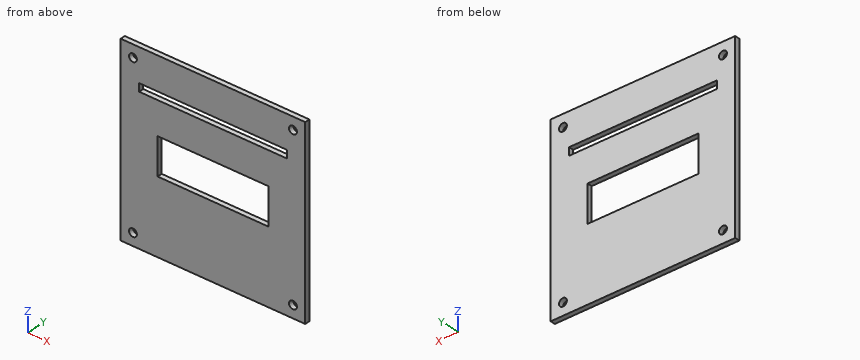
```python
from build123d import *

# Parameters (mm, degrees)
SKETCH1_W           = 75
SKETCH1_H           = 75
SKETCH1_R           = 1.6
BOSS_EXTRUDE1_DEPTH = 2
SKETCH2_W           = 45
SKETCH2_H           = 15
CUT_EXTRUDE1_DEPTH  = 10
SKETCH3_W           = 30
SKETCH3_H           = 3.2
CUT_EXTRUDE2_DEPTH  = 10


with BuildPart() as part:
    # Sketch1 → Boss-Extrude1 (new body)
    with BuildSketch(Plane(origin=(0, 0, 0), x_dir=(1, 0, 0), z_dir=(0, 1, 0))):
        Rectangle(SKETCH1_W, SKETCH1_H)
        with Locations(Location((-32.5, 32.5, 0), (0, 0, 270))):
            Circle(SKETCH1_R, mode=Mode.SUBTRACT)
        with Locations(Location((-32.5, -32.5, 0), (0, 0, 270))):
            Circle(SKETCH1_R, mode=Mode.SUBTRACT)
        with Locations(Location((32.5, 32.5, 0), (0, 0, 270))):
            Circle(SKETCH1_R, mode=Mode.SUBTRACT)
        with Locations(Location((32.5, -32.5, 0), (0, 0, 270))):
            Circle(SKETCH1_R, mode=Mode.SUBTRACT)
    extrude(amount=BOSS_EXTRUDE1_DEPTH)

    # Sketch2 → Cut-Extrude1 (cut)
    with BuildSketch(Plane.XZ):
        Rectangle(SKETCH2_W, SKETCH2_H)
    extrude(amount=-CUT_EXTRUDE1_DEPTH, mode=Mode.SUBTRACT)

    # Sketch3 → Cut-Extrude2 (cut)
    with BuildSketch(Plane.XZ):
        with Locations((-15, 22.5)):
            Rectangle(SKETCH3_W, SKETCH3_H)
        with Locations((15, 22.5)):
            Rectangle(SKETCH3_W, SKETCH3_H)
    extrude(amount=-CUT_EXTRUDE2_DEPTH, mode=Mode.SUBTRACT)


solid = part.part
```
Read the model definition and answer for the solid it produces. Units are mm, in the model's axes. Give positions to 0.01 mm unless a question says otherwise; leave off trailing zeros. Loops run counter-clockwise (first coordinate to the right, second up) from the corner with the lowest first, then second, coordinate; pieces in that order, holes last.
Item 1: Find the intervals of material crossed by line 1 along Z through (x, y) = (-22, 1.55); line 2 along X through (y, z) = (0.65, -32.5); line 3 along X through (y, z) = (1.5, 21), in increasing order.
Item 2: The part is cut by section D-D (x = 24). Write down the section's boundary in (y, z), and give its area (3 significant figures).
Item 3: The part is cut by section B-B (x = -14.5). Write down the section's boundary in (y, z), and give its area (3 significant figures).
Item 4: This flat-tipped pin is pushed along its axis until it touches: pin 1 Ø1.9 at (x, z) = (-32.5, 32.5) entering from -Y. Where does it stop, or does it pass through?
Item 5: The part is cut by section C-C (z = 32.5). Write down the section's boundary in (x, y), and give its area (3 significant figures).
Item 6: The part is cut by section A-A (z = 6). Write down the section's boundary in (x, y).
Taken from the geometry:
1. line 1: z = -37.5 to -7.5, 7.5 to 20.9, 24.1 to 37.5
1. line 2: x = -37.5 to -34.1, -30.9 to 30.9, 34.1 to 37.5
1. line 3: x = -37.5 to -30, 30 to 37.5
2. outline: (0, -37.5) - (2, -37.5) - (2, 20.9) - (0, 20.9) - close; (0, 24.1) - (2, 24.1) - (2, 37.5) - (0, 37.5) - close
2. area: 144 mm2
3. outline: (0, -37.5) - (2, -37.5) - (2, -7.5) - (0, -7.5) - close; (0, 7.5) - (2, 7.5) - (2, 20.9) - (0, 20.9) - close; (0, 24.1) - (2, 24.1) - (2, 37.5) - (0, 37.5) - close
3. area: 114 mm2
4. pin 1: passes through
5. outline: (-37.5, 0) - (-34.1, 0) - (-34.1, 2) - (-37.5, 2) - close; (-30.9, 0) - (30.9, 0) - (30.9, 2) - (-30.9, 2) - close; (34.1, 0) - (37.5, 0) - (37.5, 2) - (34.1, 2) - close
5. area: 137 mm2
6. outline: (-37.5, 0) - (-22.5, 0) - (-22.5, 2) - (-37.5, 2) - close; (22.5, 0) - (37.5, 0) - (37.5, 2) - (22.5, 2) - close
